from build123d import *

# Parameters (mm, degrees)
MAIN_BODY_DEPTH      = 1.94183
SKETCH29_R           = 5.953125
PNEUMATICMOUNT_DEPTH = 3.88366
ORINGINSERTPROFILE_W = 3.17754
ORINGINSERTPROFILE_H = 2.82448


with BuildPart() as part:
    # Sketch1 → main body (new, symmetric)
    with BuildSketch(Plane(origin=(0, 0, 0), x_dir=(1, 0, 0), z_dir=(0, 1, 0))):
        with BuildLine():
            Line((-63.5, 50.8), (-63.5, -50.8))
            ThreePointArc((-63.5, -50.8), (-59.780256121, -59.780256121), (-50.8, -63.5))
            Line((-50.8, -63.5), (50.8, -63.5))
            ThreePointArc((50.8, -63.5), (59.780256121, -59.780256121), (63.5, -50.8))
            Line((63.5, -50.8), (63.5, 50.8))
            ThreePointArc((63.5, 50.8), (59.780256121, 59.780256121), (50.8, 63.5))
            Line((50.8, 63.5), (-50.8, 63.5))
            ThreePointArc((-50.8, 63.5), (-59.780256121, 59.780256121), (-63.5, 50.8))
        make_face()
    extrude(amount=MAIN_BODY_DEPTH, both=True)

    # Sketch29 → PneumaticMount (cut)
    with BuildSketch(Plane(origin=(0, 1.94183, 0), x_dir=(1, 0, 0), z_dir=(0, 1, 0))):
        with Locations(Location((0, 0, 0), (0, 0, 270))):
            Circle(SKETCH29_R)
    extrude(amount=-PNEUMATICMOUNT_DEPTH, mode=Mode.SUBTRACT)

    # O-RingInsert: sweep along a path in ORingInsertPath
    with BuildLine(Plane(origin=(0, 1.94183, 0), x_dir=(1, 0, 0), z_dir=(0, 1, 0))) as o_ringinsert_path:
        Line((-45.992219207, -56.4388), (45.992219207, -56.4388))
        ThreePointArc((45.992219207, -56.4388), (54.972475328, -52.719056121), (58.692219207, -43.7388))
        Line((58.692219207, -43.7388), (58.692219207, 43.7388))
        ThreePointArc((58.692219207, 43.7388), (54.972475328, 52.719056121), (45.992219207, 56.4388))
        Line((45.992219207, 56.4388), (-45.992219207, 56.4388))
        ThreePointArc((-45.992219207, 56.4388), (-54.972475328, 52.719056121), (-58.692219207, 43.7388))
        Line((-58.692219207, 43.7388), (-58.692219207, -43.7388))
        ThreePointArc((-58.692219207, -43.7388), (-54.972475328, -52.719056121), (-45.992219207, -56.4388))
    # ORingInsertProfile → O-RingInsert (sweep, cut)
    with BuildSketch(Plane.XY):
        with Locations((58.692219207, 0.52959)):
            Rectangle(ORINGINSERTPROFILE_W, ORINGINSERTPROFILE_H)
    sweep(path=o_ringinsert_path.line, mode=Mode.SUBTRACT)


solid = part.part
For this review, take the finished solid that the model builds, in its own axes (mm). A direction names the side the tool comes from. Round coordinates to 2 decimals unless told otherwise and drop trailing zeros. Loops run counter-clockwise (first coordinate to the right, second up) from the corner with the lowest first, then second, coordinate; pieces in that order, holes last. Notation, with made-up numbers: (65, 75) - (74, 75) arc R26 cw to (74, 89) - close; hole circle Ø11 at (27.5, 55.5). An arc over 180 degrees is marked (long way). Use one line per item in the form item = value.
1) We need section C-C on z = 0. Write out the cut boundary in (x, y).
Solutions:
outline = (-63.5, -1.94) - (-5.95, -1.94) - (-5.95, 1.94) - (-57.1, 1.94) - (-57.1, -0.88) - (-60.28, -0.88) - (-60.28, 1.94) - (-63.5, 1.94) - close; (5.95, -1.94) - (63.5, -1.94) - (63.5, 1.94) - (60.28, 1.94) - (60.28, -0.88) - (57.1, -0.88) - (57.1, 1.94) - (5.95, 1.94) - close
2) We need section B-B on x = 0. Write out the cut boundary in (y, z), then the cut area to 3 significant figures.
Solutions:
outline = (-1.94, -63.5) - (1.94, -63.5) - (1.94, -58.03) - (-0.88, -58.03) - (-0.88, -54.85) - (1.94, -54.85) - (1.94, -5.95) - (-1.94, -5.95) - close; (-1.94, 5.95) - (1.94, 5.95) - (1.94, 54.85) - (-0.88, 54.85) - (-0.88, 58.03) - (1.94, 58.03) - (1.94, 63.5) - (-1.94, 63.5) - close
area = 429 mm2
3) We need section A-A on y = 0.8. Write out the cut boundary in (x, z), then the cut area to 3 significant figures.
Solutions:
outline = (-63.5, -50.8) arc R12.7 ccw to (-50.8, -63.5) - (50.8, -63.5) arc R12.7 ccw to (63.5, -50.8) - (63.5, 50.8) arc R12.7 ccw to (50.8, 63.5) - (-50.8, 63.5) arc R12.7 ccw to (-63.5, 50.8) - close; (-57.1, -43.74) arc R11.11 ccw to (-45.99, -54.85) - (45.99, -54.85) arc R11.11 ccw to (57.1, -43.74) - (57.1, 43.74) arc R11.11 ccw to (45.99, 54.85) - (-45.99, 54.85) arc R11.11 ccw to (-57.1, 43.74) - close; hole (-60.28, -43.74) arc R14.29 ccw to (-45.99, -58.03) - (45.99, -58.03) arc R14.29 ccw to (60.28, -43.74) - (60.28, 43.74) arc R14.29 ccw to (45.99, 58.03) - (-45.99, 58.03) arc R14.29 ccw to (-60.28, 43.74) - close; hole circle Ø11.91 at (0, 0)
area = 14,500 mm2
4) Mouldability with a two-part tool opening along X and no side actions: class faces 1 (the face through (-57.103, 1, 1)), 2 (the face through (1, 0, -63.5)), 3 (the face through (59.88, 0.03, -59.68)), 4 (the face through (55.984, 0.549, 53.953)) as pulls with the +X half, pulls with the -X half, needs draft (parallel to the pull), parting line crosses it, or undercut.
Solutions:
face_1 = undercut
face_2 = needs draft
face_3 = pulls with the +X half
face_4 = undercut
5) Wall thickness on probe 1 along X at (y, z) = (0, 0); probe 2 along Z at (x, y) = (16, 1.05); probe 3 along X at (y, z) = (0.75, 29): over which ranges is each line inside the solid? List them lowest first.
Solutions:
probe_1 = -63.5 to -60.28, -57.1 to -5.95, 5.95 to 57.1, 60.28 to 63.5
probe_2 = -63.5 to -58.03, -54.85 to 54.85, 58.03 to 63.5
probe_3 = -63.5 to -60.28, -57.1 to 57.1, 60.28 to 63.5
6) Tool access review of faces 5 (the face through (1, 1, 54.85)), 6 (the face through (59.68, 0.03, 59.88)): name each direction out of +Z, -Z, +X, -X, +Y, -Y from which nothing blocks a thin tool from reaching the whole face with its end or side.
Solutions:
face_5 = +Y
face_6 = +Z, +X, +Y, -Y
7) We need section D-D on z = 18. Write out the cut boundary in (x, y), then the cut area to 3 significant figures.
Solutions:
outline = (-63.5, -1.94) - (63.5, -1.94) - (63.5, 1.94) - (60.28, 1.94) - (60.28, -0.88) - (57.1, -0.88) - (57.1, 1.94) - (-57.1, 1.94) - (-57.1, -0.88) - (-60.28, -0.88) - (-60.28, 1.94) - (-63.5, 1.94) - close
area = 475 mm2
